For this review, take the finished solid that the model builds, in its own axes (mm). Give positions to 0.01 mm unless a question says otherwise; leave off trailing zeros. Write each loop counter-clockwise with the first axis right and the second up, starting at its lowest first coordinate (ties: lowest second). Pieces come first, ordered by that corner, then holes. Notation, with made-up numbers: M 52.5,45.5 L 71.5,45.5 A17 ccw 71.5,63.5 Z; hole C 39.25,-19.5 d1. An arc over 180 degrees is marked long. Write item = value, one per line.
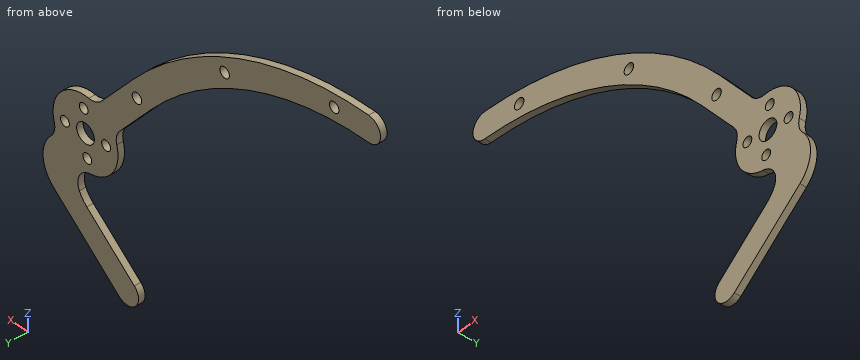
Autodesk Inventor part; units mm, degrees
ref_plane "YZ Plane" through (0, 0, 0) normal (1, 0, 0) x (0, 1, 0)
ref_plane "XZ Plane" through (0, 0, 0) normal (0, 1, 0) x (-1, 0, 0)
ref_plane "XY Plane" through (0, 0, 0) normal (0, 0, 1) x (1, 0, 0)
ref_plane "Work Plane5" through (0, 3, 0) normal (0, 1, 0) x (1, 0, 0)
sketch "Sketch2" plane through (0, 3, 0) normal (0, 1, 0) x (1, 0, 0)
  line L0 (0, 0) -> (-19.2836, -22.9813) construction
  line L1 (5.1953, 21.7488) -> (-13.9558, 37.8185) construction
  arc A0 (-95.8881, -58.7026) -> (-19.2836, -22.9813) centre (-95.8881, 41.2974) ccw construction
  line L2 (-19.2836, -22.9813) -> (-95.8881, 41.2974) construction
  line L3 (-95.8881, 41.2974) -> (-95.8881, -58.7026) construction
  line L4 (0, 0) -> (0, -11) construction
  line L5 (6.4279, 7.6604) -> (0, 0) construction
  arc A1 (6.4279, 7.6604) -> (5.1953, 21.7488) centre (-1.2326, 14.0883) ccw construction
  arc A2 (-95.8881, -54.7026) -> (-95.8881, -62.7026) centre (-95.8881, -58.7026) ccw
  arc A3 (-95.8881, -62.7026) -> (-16.2195, -25.5525) centre (-95.8881, 41.2974) ccw
  arc A4 (-95.8881, -54.7026) -> (-22.3478, -20.4102) centre (-95.8881, 41.2974) ccw
  line L6 (-19.2836, -22.9813) -> (-22.3478, -20.4102) construction
  line L7 (-19.2836, -22.9813) -> (-16.2195, -25.5525) construction
  line L8 (10.8306, 22.2418) -> (-11.3847, 40.8826)
  arc A5 (-11.3847, 40.8826) -> (-16.527, 34.7543) centre (-13.9558, 37.8185) ccw
  line L9 (-0.44, 21.2557) -> (-16.527, 34.7543)
  arc A6 (2.0873, 18.0456) -> (-0.44, 21.2557) centre (-6.8679, 13.5953) ccw
  arc A7 (12.0632, 8.1535) -> (10.8306, 22.2418) centre (4.4028, 14.5813) ccw
  circle A8 centre (0, 0) radius 7 construction
  arc A9 (-1.1061, -10.9442) -> (10.5859, 2.9897) centre (0, 0) ccw
  arc A10 (-1.6433, 10.8766) -> (-10.5859, -2.9897) centre (0, 0) ccw
  line L10 (-16.2195, -25.5525) -> (-5.4391, -12.705)
  line L11 (11.5675, 7.5627) -> (12.0632, 8.1535)
  line L12 (-22.3478, -20.4102) -> (-11.5675, -7.5627)
  arc A11 (-1.1061, -10.9442) -> (-5.4391, -12.705) centre (-1.6089, -15.9189) ccw
  arc A12 (11.5675, 7.5627) -> (10.5859, 2.9897) centre (15.3977, 4.3487) ccw
  arc A13 (-11.5675, -7.5627) -> (-10.5859, -2.9897) centre (-15.3977, -4.3487) ccw
  arc A14 (-1.6433, 10.8766) -> (2.0873, 18.0456) centre (-2.3903, 15.8204) ccw
  circle A15 centre (0, 0) radius 3
  circle A16 centre (-6.9734, -0.6101) radius 1.5
  line L13 (0, 0) -> (-6.9734, -0.6101) construction
  circle A17 centre (0.6101, -6.9734) radius 1.5
  circle A18 centre (6.9734, 0.6101) radius 1.5
  circle A19 centre (-0.6101, 6.9734) radius 1.5
  point P0 (12.8558, 15.3209)
  point P1 (-3.5224, -10.4208)
  point P2 (9.6508, 5.2785)
  dimension "d53" = 14
  dimension "d24" = 30
  dimension "d27" = 35
  dimension "d28" = 20
  dimension "d29" = 100
  dimension "d30" = 50
  dimension "d41" = 10
  dimension "d42" = 140
  dimension "d50" = 8
  dimension "d51" = 4
  dimension "d52" = 10
  dimension "d55" = 11
  dimension "d56" = 11
  dimension "d57" = 5
  dimension "d58" = 6
  dimension "d62" = 3
  dimension "d63" = 45
  dimension "d66" = 360
extrude "Extrusion2" add sketch "Sketch2" along normal blind 2
sketch "Sketch4" plane through (0, 5, 0) normal (0, 1, 0) x (1, 0, 0)
  arc A0 (-95.8881, -54.7026) -> (-22.3478, -20.4102) centre (-95.8881, 41.2974) ccw construction
  arc A1 (-84.2223, -58.0198) -> (-17.4113, -20.6815) centre (-95.8881, 41.2974) ccw construction
  line L0 (-84.2223, -58.0198) -> (-95.8881, 41.2974) construction
  line L1 (-95.8881, 41.2974) -> (-17.4113, -20.6815) construction
  circle A2 centre (0, 0) radius 3 construction
  line L2 (-95.8881, 41.2974) -> (0, 0) construction
  point P0 (-47.1033, -45.9954)
  dimension "d68" = 4
  dimension "d69" = 45
  dimension "d70" = 15
hole "Hole1" at (-84.2223, 5, 58.0198) at (-47.1033, 5, 45.9954) at (-17.4113, 5, 20.6815) direction (0, -1, 0) diameter 3.2 end through all
sketch "Sketch5" plane through (0, 5, 0) normal (0, 1, 0) x (1, 0, 0)
  circle A0 centre (-47.1033, -45.9954) radius 1.6
  circle A1 centre (-84.2223, -58.0198) radius 1.6
  circle A2 centre (-17.4113, -20.6815) radius 1.6
  circle A3 centre (0, 0) radius 3
  circle A4 centre (-0.6101, 6.9734) radius 1.5
  circle A5 centre (6.9734, 0.6101) radius 1.5
  circle A6 centre (0.6101, -6.9734) radius 1.5
  circle A7 centre (-6.9734, -0.6101) radius 1.5
  arc A8 (-95.8881, -62.7026) -> (-16.2195, -25.5525) centre (-95.8881, 41.2974) ccw
  line L0 (-16.2195, -25.5525) -> (-5.4391, -12.705)
  arc A9 (-1.1061, -10.9442) -> (-5.4391, -12.705) centre (-1.6089, -15.9189) ccw
  arc A10 (-1.1061, -10.9442) -> (10.5859, 2.9897) centre (0, 0) ccw
  arc A11 (11.5675, 7.5627) -> (10.5859, 2.9897) centre (15.3977, 4.3487) ccw
  line L1 (11.5675, 7.5627) -> (12.0632, 8.1535)
  arc A12 (12.0632, 8.1535) -> (10.8306, 22.2418) centre (4.4028, 14.5813) ccw
  line L2 (10.8306, 22.2418) -> (-11.3847, 40.8826)
  arc A13 (-11.3847, 40.8826) -> (-16.527, 34.7543) centre (-13.9558, 37.8185) ccw
  line L3 (-16.527, 34.7543) -> (-0.44, 21.2557)
  arc A14 (2.0873, 18.0456) -> (-0.44, 21.2557) centre (-6.8679, 13.5953) ccw
  arc A15 (-1.6433, 10.8766) -> (2.0873, 18.0456) centre (-2.3903, 15.8204) ccw
  arc A16 (-1.6433, 10.8766) -> (-10.5859, -2.9897) centre (0, 0) ccw
  arc A17 (-11.5675, -7.5627) -> (-10.5859, -2.9897) centre (-15.3977, -4.3487) ccw
  line L4 (-11.5675, -7.5627) -> (-22.3478, -20.4102)
  arc A18 (-95.8881, -54.7026) -> (-22.3478, -20.4102) centre (-95.8881, 41.2974) ccw
  arc A19 (-95.8881, -54.7026) -> (-95.8881, -62.7026) centre (-95.8881, -58.7026) ccw
properties part number "wstepna_geometria_wersja_2"
1. We need section B-B, the plane z = -16. Write out the cut boundary in (x, y).
Responses:
outline = M 2.61,3 L 14.3,3 L 14.3,5 L 2.61,5 Z
2. Insertion check: P1, Ø4, axis at x = -17.41, z = 20.68, coming from the +Y side; P2, Ø2.5, axis at x = -47.1, z = 46, coming from the -Y side. Each pin has a flat end and moves straight along its axis. Give the tip position at first contact, or say it passes through.
Responses:
P1 = 5
P2 = through
3. We need section A-A, the plane y = 4.45. Count the separate pieces of the cut face and the enclosed holes in it, then the cut area to 3 significant figures.
Responses:
separate_pieces = 1
enclosed_holes = 8
area = 1,570 mm2
4. For line 1 along Z through (x, y) = (0, 3.5); line 2 along Z through (x, y) = (-7.5, 3.45); line 3 along X through (y, z) = (3.6, -20), list the stretches that pass through material, from the lowest coordinate up. Write a range as from..to.
Responses:
line_1 = -31.33..-20.86, -11.43..-8.34, -5.6..-3, 3..5.6, 8.34..11
line_2 = -37.62..-27.18, -8.05..-0.79, 2.01..15.16
line_3 = 0.81..12.81
5. We need section C-C, the plane x = -71.5. Write out the cut boundary in (y, z).
Responses:
outline = M 3,51.55 L 5,51.55 L 5,59.8 L 3,59.8 Z
